from build123d import *

# Parameters (mm, degrees)
SKETCH1_R           = 88.9
BOSS_EXTRUDE1_DEPTH = 3
CUT_EXTRUDE2_DEPTH  = 3


with BuildPart() as part:
    # Sketch1 → Boss-Extrude1 (new body)
    with BuildSketch(Plane(origin=(0, 0, 0), x_dir=(1, 0, 0), z_dir=(0, 1, 0))):
        with Locations(Location((0, 0, 0), (0, 0, 270))):
            Circle(SKETCH1_R)
    extrude(amount=BOSS_EXTRUDE1_DEPTH)

    # Sketch3 → Cut-Extrude2 (cut)
    with BuildSketch(Plane.XZ):
        with BuildLine():
            Line((53, -41), (-53, -41))
            ThreePointArc((-53, -41), (-55.828427125, -39.828427125), (-57, -37))
            Line((-57, -37), (-57, 37))
            ThreePointArc((-57, 37), (-55.828427125, 39.828427125), (-53, 41))
            Line((-53, 41), (53, 41))
            ThreePointArc((53, 41), (55.828427125, 39.828427125), (57, 37))
            Line((57, 37), (57, -37))
            ThreePointArc((57, -37), (55.828427125, -39.828427125), (53, -41))
        make_face()
    extrude(amount=-CUT_EXTRUDE2_DEPTH, mode=Mode.SUBTRACT)


solid = part.part
Source: CAD feature listing. Evaluate the final solid. Frame: model axes, mm. A direction names the side the tool comes from. Round coordinates to 2 decimals unless told otherwise and drop trailing zeros. Write each loop counter-clockwise with the first axis right and the second up, starting at its lowest first coordinate (ties: lowest second). Pieces come first, ordered by that corner, then holes. Notation, with made-up numbers: M -25.75,24.5 L 12.25,24.5 A23 cw 12.25,36.5 Z; hole C 1.5,81.5 d4. An arc over 180 degrees is marked long. One line per item, written item: value. Start each with the question number.
Item 1: Ray query, L1, parallel to X at y = 1.15, z = -0.5; L2, parallel to Z at x = 38.5, y = 1.85; L3, parallel to X at y = 2.45, z = -21. Return the intervals inside material, ascending. Write a range as from..to.
Item 2: Section query B-B (z = 0). Return the cut outline in (x, y).
Item 3: Pin query (flat end, axial travel): pin 1 (0.9 mm diameter, centred on y = 1.5, z = -17.5, fed in from -X). Return the tip coordinate at first contact, or that it passes through.
Item 4: Set-up query: faces 5 (the flat face through (-58, 0, -1)), 6 (the cylindrical face through (55.797, 1.479, 39.859)). Return all of +Z, -Z, +X, -X, +Y, -Y with unobstructed straight access to the full face (end or side cutting, diameter ignored); none if empty.
Item 5: Mould query, pull axis X, two halves, no side actions, for faces 1 (the cylindrical face through (-55.797, 1.479, -39.859)), 2 (the cylindrical face through (74.96, 1.48, 47.79)), 3 (the flat face through (-58, 3, -1)), 4 (the cylindrical face through (-55.859, 1.479, 39.797)). Classes: pulls with the +X half, pulls with the -X half, needs draft (parallel to the pull), parting line crosses it, or undercut.
Item 6: Section query C-C (y = 1.45). Return the cut outline in (x, z), plus the area to 3 significant figures.
Item 7: Section query D-D (z = 45). Return the cut outline in (x, y), plus the area to 3 significant figures.
Item 8: Section query A-A (x = 0). Return the cut outline in (y, z).
Result set:
1. L1: x = -88.9..-57, 57..88.9
1. L2: z = -80.13..-41, 41..80.13
1. L3: x = -86.38..-57, 57..86.38
2. outline: M -88.9,0 L -57,0 L -57,3 L -88.9,3 Z; M 57,0 L 88.9,0 L 88.9,3 L 57,3 Z
3. pin 1: stops at x = -87.25
4. face 5: +Z, -Z, +X, -X, -Y
4. face 6: +Y, -Y
5. face 1: undercut
5. face 2: parting line crosses it
5. face 3: needs draft
5. face 4: undercut
6. outline: C 0,0 d177.8; hole M -57,-37 A4 ccw -53,-41 L 53,-41 A4 ccw 57,-37 L 57,37 A4 ccw 53,41 L -53,41 A4 ccw -57,37 Z
6. area: 15,500 mm²
7. outline: M -76.67,0 L 76.67,0 L 76.67,3 L -76.67,3 Z
7. area: 460 mm²
8. outline: M 0,-88.9 L 3,-88.9 L 3,-41 L 0,-41 Z; M 0,41 L 3,41 L 3,88.9 L 0,88.9 Z
